Design review of the part shown in the three views and the two pictorial views. Dimensions are in mm from the part's minimum x, y and z. A direction names the side the tool comes from. Round coordinates to 2 decimals unless told otherwise and drop trailing zeros. Order: outer loops, then holes, each group sorted by start corner. A loop starts at its lowest first (then second) coordinate and runs counter-clockwise, first axis right, second up. Notation, with made-up numbers: (89, 42) - (139, 42) arc R13 ccw to (139, 61) - close; hole circle Ø2 at (81.25, 2.25). An arc over 180 degrees is marked (long way). One line per item, written item: value.
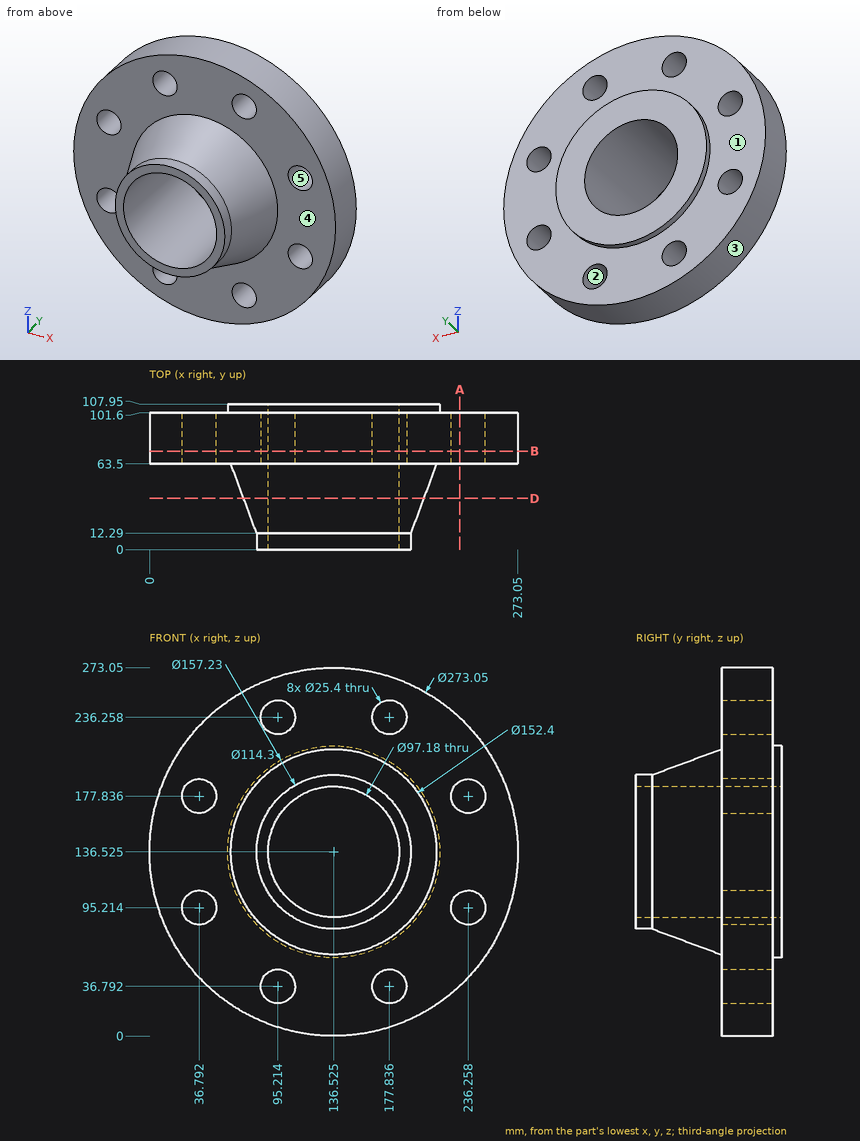
Item 1: Machinability: for the marked faces 1 and 2, which of the approach directions +Z, -Z, +X, -X, +Y, -Y give a long, thin tool a straight path to every point of the face, cutting with its end or side? Answer none if there is none.
Returned:
face 1: +Y
face 2: +Y, -Y
Item 2: Take a section at B-B (y = 73). Count the separate pieces of the cut face and the enclosed holes in it, plus the area to 3 significant figures.
Returned:
separate pieces: 1
enclosed holes: 9
area: 47,100 mm^2
Item 3: For P1, Ø23, axis at x = 177.84, z = 236.26, coming from the -Y side; P2, Ø3, axis at x = 118, y = 79.5, coming from the +Z side; P3, Ø8, axis at x = 79.5, y = 60, coming from the -Z side; P4, Ø6, axis at y = 36, z = 185.5, coming from the -X side (1 decimal), all flat-tipped, find the tip position at first contact; note any pin that passes through.
Returned:
P1: through
P2: z = 271.98
P3: z = 11.61
P4: x = 88.8
Item 4: Wall thickness on line 1 (Y direction, x = 164.5, z = 258.5); line 2 (X direction, y = 59, z = 127); line 3 (Z direction, x = 112, y = 63) (1 decimal): over which ranges is each line inside the solid? List them lowest first.
Returned:
line 1: 63.5 to 101.6
line 2: 62.61 to 88.88, 184.17 to 210.44
line 3: 64.6 to 94.6, 178.5 to 208.5
Item 5: Take a section at A-A (x = 230). Write out the cut boundary in (y, z) (1 decimal).
Returned:
outline: (63.5, 37) - (101.6, 37) - (101.6, 84.2) - (63.5, 84.2) - close; (63.5, 106.3) - (101.6, 106.3) - (101.6, 166.8) - (63.5, 166.8) - close; (63.5, 188.9) - (101.6, 188.9) - (101.6, 236) - (63.5, 236) - close
Item 6: Take a section at D-D (y = 38). Write out the cut boundary in (x, z) (1 decimal).
Returned:
outline: circle Ø133.4 at (136.5, 136.5); hole circle Ø97.2 at (136.5, 136.5)
Item 7: The part is to be moulded in two halves that separate along Z. For the marked faces 3, 4 and 5, say which applies: +Z half, -Z half, draft (parallel to the pull), parting line (faces both ways), or undercut.
Returned:
face 3: parting line
face 4: draft
face 5: undercut
